Job drawing, mm, ordinate dimensions from the low corner. One solid piece. A direction names the side the tool comes from. Give positions to 0.01 mm unless a question says otherwise; leave off trailing zeros. Write each loop counter-clockwise with the first axis right and the second up, starting at its lowest first coordinate (ties: lowest second). Pieces come first, ordered by that corner, then holes. Notation, with made-up numbers: M -6.75,79 L 28.25,79 A18 cw 28.25,107 Z; hole C 4.5,-25.75 d3. An arc over 180 degrees is marked long. Use a Markdown table: item, result.
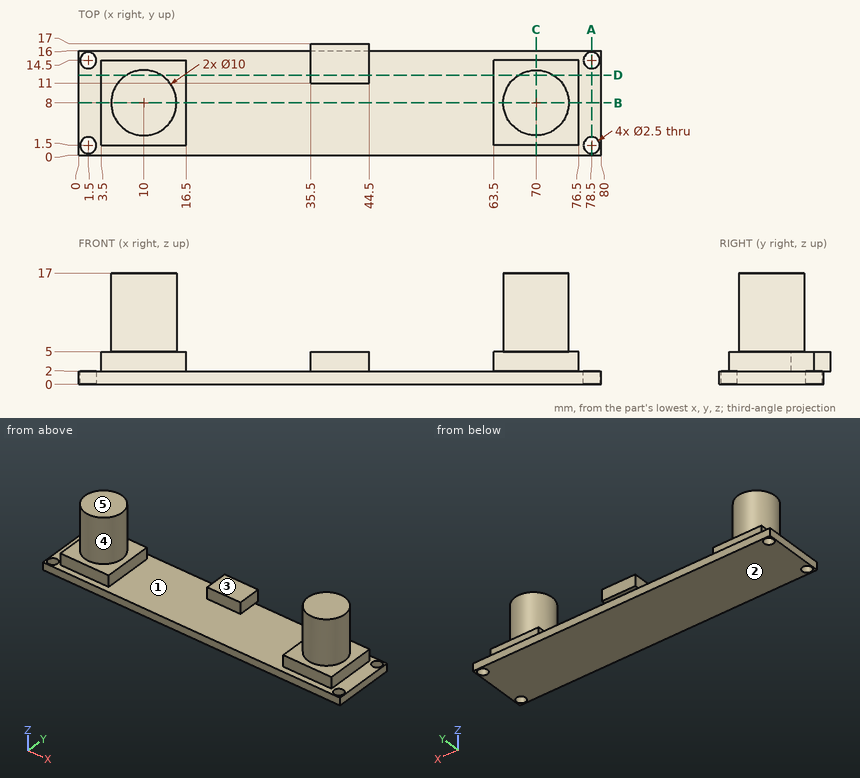
1. Cut at B-B, the plane y = 8. Give the cut face in (x, z).
Findings below:
| item | result |
|---|---|
| outline | M 0,0 L 80,0 L 80,2 L 76.5,2 L 76.5,5 L 75,5 L 75,17 L 65,17 L 65,5 L 63.5,5 L 63.5,2 L 16.5,2 L 16.5,5 L 15,5 L 15,17 L 5,17 L 5,5 L 3.5,5 L 3.5,2 L 0,2 Z |
2. Drill centre lines: L1, parallel to Y at x = 1.5, z = 1.55; L2, parallel to X at y = 8, z = 10; L3, parallel to Z at x = 47, y = 15.25. Where is each one in solid material? Low to high.
Findings below:
| item | result |
|---|---|
| L1 | 0 to 0.25, 2.75 to 13.25, 15.75 to 16 |
| L2 | 5 to 15, 65 to 75 |
| L3 | 0 to 2 |
3. Tool access for the marked faces 3, 4 and 5: list every direction of +Z, -Z, +X, -X, +Y, -Y with a clear straight run to the whole face (end or side of a thin tool).
Findings below:
| item | result |
|---|---|
| face 3 | +Z, +Y, -Y |
| face 4 | +Z |
| face 5 | +Z, +X, -X, +Y, -Y |
4. Cut at C-C, the plane x = 70. Give the cut face in (y, z), then the cut area to 3 significant figures.
Findings below:
| item | result |
|---|---|
| outline | M 0,0 L 16,0 L 16,2 L 14.5,2 L 14.5,5 L 13,5 L 13,17 L 3,17 L 3,5 L 1.5,5 L 1.5,2 L 0,2 Z |
| area | 191 mm2 |
5. Drop flat-ended pins along their axis: P1, Ø1.5, axis at x = 36.5, z = 7, coming from the +Y side; P2, Ø3, axis at x = 78.5, y = 14.5, coming from the +Z side; P3, Ø8, axis at y = 12, z = 6.5, coming from the -X side; P4, Ø0.9, axis at x = 10.5, z = 3, coming from the -Y side. Give the stop position or say it passes through.
Findings below:
| item | result |
|---|---|
| P1 | through |
| P2 | z = 2 |
| P3 | x = 3.5 |
| P4 | y = 1.5 |
6. Two-plate mould, pull along X, no slides. Class the marked faces 1 and 2: released by +X, released by -X, zero draft, split by the parting line, or undercut.
Findings below:
| item | result |
|---|---|
| face 1 | undercut |
| face 2 | zero draft |
7. Cut at A-A, the plane x = 78.5. Give the cut face in (y, z).
Findings below:
| item | result |
|---|---|
| outline | M 0,0 L 0.25,0 L 0.25,2 L 0,2 Z; M 2.75,0 L 13.25,0 L 13.25,2 L 2.75,2 Z; M 15.75,0 L 16,0 L 16,2 L 15.75,2 Z |
8. Cut at D-D, the plane y = 12.25. Give the cut face in (x, z), then the cut area to 3 significant figures.
Findings below:
| item | result |
|---|---|
| outline | M 0,0 L 80,0 L 80,2 L 76.5,2 L 76.5,5 L 72.63,5 L 72.63,17 L 67.37,17 L 67.37,5 L 63.5,5 L 63.5,2 L 44.5,2 L 44.5,5 L 35.5,5 L 35.5,2 L 16.5,2 L 16.5,5 L 12.63,5 L 12.63,17 L 7.37,17 L 7.37,5 L 3.5,5 L 3.5,2 L 0,2 Z |
| area | 391 mm2 |
